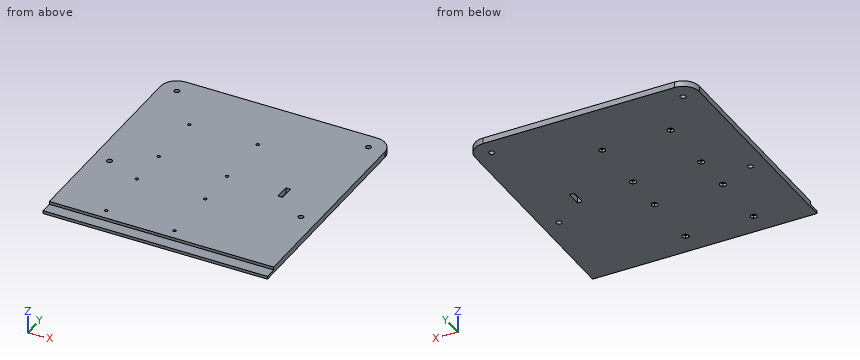
```python
from build123d import *

# Parameters (mm, degrees)
SKETCH4_R           = 2.25
SKETCH4_R_2         = 7.9375
BOSS_EXTRUDE1_DEPTH = 5
CUT_EXTRUDE1_DEPTH  = 191.5
SKETCH8_R           = 1.35
SKETCH8_R_2         = 1.3
CUT_EXTRUDE2_DEPTH  = 6
SKETCH9_R           = 1.35
SKETCH9_R_2         = 1.3
CUT_EXTRUDE3_DEPTH  = 6
CUT_EXTRUDE4_DEPTH  = 2.4
SKETCH12_W          = 4
SKETCH12_H          = 12.7
CUT_EXTRUDE5_DEPTH  = 6


with BuildPart() as part:
    # Sketch4 → Boss-Extrude1 (new body)
    with BuildSketch(Plane.XY):
        with BuildLine():
            Line((-66.080112923, -1201.56262), (96.419887077, -1201.56262))
            ThreePointArc((96.419887077, -1201.56262), (106.319382013, -1197.462114937), (110.419887077, -1187.56262))
            Line((110.419887077, -1187.56262), (110.419887077, -812.43738))
            ThreePointArc((110.419887077, -812.43738), (106.319382013, -802.537885063), (96.419887077, -798.43738))
            Line((96.419887077, -798.43738), (-66.080112923, -798.43738))
            ThreePointArc((-66.080112923, -798.43738), (-75.97960786, -802.537885063), (-80.080112923, -812.43738))
            Line((-80.080112923, -812.43738), (-80.080112923, -1187.56262))
            ThreePointArc((-80.080112923, -1187.56262), (-75.97960786, -1197.462114937), (-66.080112923, -1201.56262))
        make_face()
        with Locations((96.419887077, -1080)):
            Circle(SKETCH4_R, mode=Mode.SUBTRACT)
        with Locations((88.147808187, -1029.0799835)):
            Circle(SKETCH4_R_2, mode=Mode.SUBTRACT)
        with Locations((-66.080112923, -1080)):
            Circle(SKETCH4_R, mode=Mode.SUBTRACT)
        with Locations((96.419887077, -920)):
            Circle(SKETCH4_R, mode=Mode.SUBTRACT)
        with Locations((-66.080112923, -920)):
            Circle(SKETCH4_R, mode=Mode.SUBTRACT)
        with Locations((-66.080112923, -1187.56262)):
            Circle(SKETCH4_R, mode=Mode.SUBTRACT)
        with Locations((96.419887077, -1187.56262)):
            Circle(SKETCH4_R, mode=Mode.SUBTRACT)
        with Locations((-66.080112923, -812.43738)):
            Circle(SKETCH4_R, mode=Mode.SUBTRACT)
        with Locations((96.419887077, -812.43738)):
            Circle(SKETCH4_R, mode=Mode.SUBTRACT)
    extrude(amount=BOSS_EXTRUDE1_DEPTH)

    # Sketch5 → Cut-Extrude1 (cut, through all)
    with BuildSketch(Plane(origin=(110.419887077, 0, 0), x_dir=(0, 0, -1), z_dir=(1, 0, 0))):
        Polygon((-2.5, -990), (-2.5, -1000), (0, -1000), (105.330135386, -1133.485190723), (-31.100407904, -1241.139436993), (-117.784745415, -1052.296655995), (-5, -990), align=None)
    extrude(amount=-CUT_EXTRUDE1_DEPTH, mode=Mode.SUBTRACT)

    # Sketch8 → Cut-Extrude2 (cut, through all)
    with BuildSketch(Plane(origin=(0, 0, 0), x_dir=(1, 0, 0), z_dir=(0, 0, -1))):
        with Locations((-36.405274736, 897.30672742)):
            Circle(SKETCH8_R)
        with Locations((21.594725264, 897.30672742)):
            Circle(SKETCH8_R)
        with Locations((21.594725264, 848.30672742)):
            Circle(SKETCH8_R)
        with Locations((-36.405274736, 848.30672742)):
            Circle(SKETCH8_R_2)
    extrude(amount=-CUT_EXTRUDE2_DEPTH, mode=Mode.SUBTRACT)

    # Sketch9 → Cut-Extrude3 (cut, through all)
    with BuildSketch(Plane(origin=(0, 0, 0), x_dir=(1, 0, 0), z_dir=(0, 0, -1))):
        with Locations((-36.451263927, 981.041793441)):
            Circle(SKETCH9_R)
        with Locations((21.548736073, 981.041793441)):
            Circle(SKETCH9_R)
        with Locations((21.548736073, 932.041793441)):
            Circle(SKETCH9_R)
        with Locations((-36.451263927, 932.041793441)):
            Circle(SKETCH9_R_2)
    extrude(amount=-CUT_EXTRUDE3_DEPTH, mode=Mode.SUBTRACT)

    # Sketch11 → Cut-Extrude4 (cut)
    with BuildSketch(Plane(origin=(0, 0, 0), x_dir=(-1, 0, 0), z_dir=(0, 0, -1))):
        Polygon((-20.122482078, -845.75672742), (-23.066968451, -845.75672742), (-24.539211637, -848.30672742), (-23.066968451, -850.85672742), (-20.122482078, -850.85672742), (-18.650238891, -848.30672742), align=None)
        Polygon((34.933031549, -845.75672742), (33.460788363, -848.30672742), (34.933031549, -850.85672742), (37.877517922, -850.85672742), (39.349761109, -848.30672742), (37.877517922, -845.75672742), align=None)
        Polygon((34.933031549, -894.75672742), (33.460788363, -897.30672742), (34.933031549, -899.85672742), (37.877517922, -899.85672742), (39.349761109, -897.30672742), (37.877517922, -894.75672742), align=None)
        Polygon((-20.122482078, -894.75672742), (-23.066968451, -894.75672742), (-24.539211637, -897.30672742), (-23.066968451, -899.85672742), (-20.122482078, -899.85672742), (-18.650238891, -897.30672742), align=None)
        Polygon((-20.076492886, -929.491793441), (-23.020979259, -929.491793441), (-24.493222445, -932.041793441), (-23.020979259, -934.591793441), (-20.076492886, -934.591793441), (-18.6042497, -932.041793441), align=None)
        Polygon((34.979020741, -929.491793441), (33.506777555, -932.041793441), (34.979020741, -934.591793441), (37.923507114, -934.591793441), (39.3957503, -932.041793441), (37.923507114, -929.491793441), align=None)
        Polygon((-23.020979259, -978.491793441), (-24.493222445, -981.041793441), (-23.020979259, -983.591793441), (-20.076492886, -983.591793441), (-18.6042497, -981.041793441), (-20.076492886, -978.491793441), align=None)
        Polygon((34.979020741, -978.491793441), (33.506777555, -981.041793441), (34.979020741, -983.591793441), (37.923507114, -983.591793441), (39.3957503, -981.041793441), (37.923507114, -978.491793441), align=None)
    extrude(amount=-CUT_EXTRUDE4_DEPTH, mode=Mode.SUBTRACT)

    # Sketch12 → Cut-Extrude5 (cut, through all)
    with BuildSketch(Plane.XY.offset(5)):
        with Locations((69.759334594, -896.65140708)):
            Rectangle(SKETCH12_W, SKETCH12_H)
    extrude(amount=-CUT_EXTRUDE5_DEPTH, mode=Mode.SUBTRACT)


solid = part.part
```
Could you check a few things on this model? Use its own coordinates, in mm. Round coordinates to 2 decimals unless told otherwise and drop trailing zeros. Write each loop counter-clockwise with the first axis right and the second up, starting at its lowest first coordinate (ties: lowest second). Pieces come first, ordered by that corner, then holes. Notation, with made-up numbers: M -25,26.5 L 15,26.5 A32 ccw 15,61.5 Z; hole C 53.25,-30.5 d10. An arc over 180 degrees is marked long. Answer in a Markdown table with one row per item. Add a question column.
Q1. Will this pin go through, and if not, where does the flat tip stop? pin 1 Ø2.5 at (x, y) = (-37, -897) entering from -Z.
Q2. Imagine slicing it at C-C (x = -23.5). Please give me the cut outline in (y, z).
Q3. Imagine slicing it at B-B (z = 3.9). Give the number of separate pieces and of enclosed holes in the cut face, then the cut area to 3 significant figures.
Q4. If I drill on line 1 (X direction, y = -848, z = 3.5); line 2 (X direction, y = -894, z = 3.75); line 3 (Y direction, x = 95, z = 0.65), over which ranges is the centre line in solid material (lowest first)? Write a range as from..to.
Q5. Imagine slicing it at A-A (y = -920). Please give me the cut outline in (x, z).
Values:
| question | item | result |
|---|---|---|
| 1 | pin 1 | z = 2.4 |
| 2 | outline | M -1000,0 L -798.44,0 L -798.44,5 L -990,5 L -990,2.5 L -1000,2.5 Z |
| 3 | separate pieces | 1 |
| 3 | enclosed holes | 13 |
| 3 | area | 36,200 mm^2 |
| 4 | line 1 | -80.08..-37.67, -35.14..20.28, 22.91..110.42 |
| 4 | line 2 | -80.08..67.76, 71.76..110.42 |
| 4 | line 3 | -1000..-921.75, -918.25..-814.18, -810.69..-798.44 |
| 5 | outline | M -80.08,0 L -68.33,0 L -68.33,5 L -80.08,5 Z; M -63.83,0 L 94.17,0 L 94.17,5 L -63.83,5 Z; M 98.67,0 L 110.42,0 L 110.42,5 L 98.67,5 Z |
